```python
from build123d import *

# Parameters (mm, degrees)
F1_DEPTH = 25.4
F2_R     = 6.35
F3_W     = 65.815818
F3_H     = 34.738873
F4_DEPTH = 15.774595
F5_W     = 13.649403
F5_H     = 52.52206
F6_DEPTH = 22.861
F7_W     = 3.175
F7_H     = 6.35
F8_DEPTH = 1.27


with BuildPart() as f1:
    # F0 (on Top) → F1 (new body)
    with BuildSketch(Plane.XY):
        with BuildLine():
            Line((-3.073595, 27.77132), (-3.073595, -27.77132))
            ThreePointArc((-3.073595, -27.77132), (-0.770738, -13.970444), (0, 0))
            ThreePointArc((0, 0), (-0.770738, 13.970444), (-3.073595, 27.77132))
        make_face()
        Polygon((-15.773595, -27.599099), (-3.073595, -27.77132), (-3.073595, 27.77132), (-15.773595, 27.599099), align=None)
    extrude(amount=F1_DEPTH)

    # F2
    f2_edges = [f1.edges().sort_by_distance(p)[0] for p in [
        (-3.073595, 27.77132, 12.7),
        (-3.073595, -27.77132, 12.7),
    ]]
    fillet(f2_edges, radius=F2_R)

    # F3 (on Right) → F4 (cut, through all)
    with BuildSketch(Plane.YZ):
        with Locations((2.774937, 10.382003)):
            Rectangle(F3_W, F3_H)
        Polygon((-12.7, 10.16), (-12.7, 22.86), (12.7, 22.86), (12.7, 10.16), (24.13, 10.16), (24.13, 3.81), (-24.13, 3.81), (-24.13, 10.16), align=None, mode=Mode.SUBTRACT)
    extrude(amount=-F4_DEPTH, mode=Mode.SUBTRACT)

    # F5 (on Top) → F6 (cut, through all)
    with BuildSketch(Plane.XY):
        with Locations((-9.872701, -0.828976)):
            Rectangle(F5_W, F5_H)
    extrude(amount=F6_DEPTH, mode=Mode.SUBTRACT)

    # F7 (on Right) → F8 (cut)
    with BuildSketch(Plane.YZ):
        with Locations((-3.175, 14.605)):
            Rectangle(F7_W, F7_H)
        with Locations((3.175, 14.605)):
            Rectangle(F7_W, F7_H)
    extrude(amount=-F8_DEPTH, mode=Mode.SUBTRACT)


solid = f1.part
```
The model under review builds one solid part; all positions refer to its coordinate system, in mm. A direction names the side the tool comes from. Give positions to 0.01 mm unless a question says otherwise; leave off trailing zeros. Order: outer loops, then holes, each group sorted by start corner. A loop starts at its lowest first (then second) coordinate and runs counter-clockwise, first axis right, second up. Notation, with made-up numbers: (-16.75, 60.25) - (30.25, 60.25) arc R19 ccw to (30.25, 68.25) - close; hole circle Ø11 at (-10.75, -8.5). An arc over 180 degrees is marked (long way). Use CSV: the item, a comma, the result in double quotes. Start each with the question number.
Q1. Tool access review of faces 5 (the flat face through (-2, 17, 10.16)), 6 (the flat face through (-1, -3, 17.78)), 7 (the flat face through (-2, -12.7, 16)): name each direction out of +Z, -Z, +X, -X, +Y, -Y from which nothing blocks a thin tool from reaching the whole face with its end or side.
Q2. Clearance check with flat-ended pins moving along their axes: pin 1 Ø1.2 at (x, y) = (-2.5, -18.5) entering from +Z; pin 2 Ø1.2 at (x, z) = (-1.5, 16) entering from -Y; pin 3 Ø1.2 at (x, z) = (-2.5, 19) entering from +Y. State where each tip first meets the part, or that it passes through.
Q3. The part is to be moulded in two halves that separate along Z. For faces 1 (the flat face through (-2, 0, 3.81)), 2 (the flat face through (-3.048, 0, 11)), 3 (the flat face through (-2, -17, 10.16)), 4 (the flat face through (-1, 1.588, 15)), say which applies: +Z half, -Z half, draft (parallel to the pull), parting line (faces both ways), or undercut.
Q4. To check wall thickness, follow line 1 along Z through (x, y) = (-0.15, 2); line 2 along Z through (x, y) = (-1.55, 14); line 3 along X through (y, z) = (0.5, 20.5). State the ranges of each line that lie inside material, in increasing order. Write a range as [from, to].
Q5. We need section A-A, the plane z = 12. Write out the cut boundary in (x, y), and give its area (3 significant figures).
Q6. We need section C-C, the plane y = -16. Write out the cut boundary in (x, z).
Q7. We need section D-D, the plane z = 21.25. Write out the cut boundary in (x, y), and give its area (3 significant figures).
Q8. We need section B-B, the plane z = 9.5. Write out the cut boundary in (x, y), and give its area (3 significant figures).
Outcome:
1,face 5,"+Z, +X, -X, +Y"
1,face 6,"+X"
1,face 7,"+Z, +X, -X, -Y"
2,pin 1,"stops at z = 10.16"
2,pin 2,"stops at y = -12.7"
2,pin 3,"stops at y = 12.7"
3,face 1,"-Z half"
3,face 2,"draft"
3,face 3,"+Z half"
3,face 4,"undercut"
4,line 1,"z = [3.81, 11.43], [17.78, 22.86]"
4,line 2,"z = [3.81, 10.16]"
4,line 3,"x = [-3.05, 0]"
5,outline,"(-3.05, -12.7) - (-0.64, -12.7) arc R127 ccw to (-0.09, -4.76) - (-1.27, -4.76) - (-1.27, -1.59) - (-0.01, -1.59) arc R127 ccw to (0, 0) arc R127 ccw to (-0.01, 1.59) - (-1.27, 1.59) - (-1.27, 4.76) - (-0.09, 4.76) arc R127 ccw to (-0.64, 12.7) - (-3.05, 12.7) - close"
5,area,"64.2 mm^2"
6,outline,"(-3.05, 3.81) - (-1.01, 3.81) - (-1.01, 10.16) - (-3.05, 10.16) - close"
7,outline,"(-3.05, -12.7) - (-0.64, -12.7) arc R127 ccw to (0, 0) arc R127 ccw to (-0.64, 12.7) - (-3.05, 12.7) - close"
7,area,"72.0 mm^2"
8,outline,"(-3.05, -24.13) - (-2.54, -24.13) arc R6.35 ccw to (-2, -22.47) arc R127 ccw to (0, 0) arc R127 ccw to (-2, 22.47) arc R6.35 ccw to (-2.54, 24.13) - (-3.05, 24.13) - close"
8,area,"110 mm^2"
